Verification items for the finished model (mm, model axes). Face numbers are marked on the shaded views. Round coordinates to 2 decimals unless told otherwise and drop trailing zeros. Loops run counter-clockwise (first coordinate to the right, second up) from the corner with the lowest first, then second, coordinate; pieces in that order, holes last. Notation, with made-up numbers: M -21.5,-28 L 37.5,-28 A20 ccw 37.5,-4 Z; hole C 43.25,12.5 d5. An arc over 180 degrees is marked long. One line per item, written item: value.
Autodesk Inventor part; units mm, degrees
ref_plane "YZ Plane" through (0, 0, 0) normal (1, 0, 0) x (0, 1, 0)
ref_plane "XZ Plane" through (0, 0, 0) normal (0, 1, 0) x (-1, 0, 0)
ref_plane "XY Plane" through (0, 0, 0) normal (0, 0, 1) x (1, 0, 0)
sketch "Sketch1" plane through (0, 0, 0) normal (0, 1, 0) x (-1, 0, 0)
  line L0 (0, 0) -> (114.8965, 0) construction
  line L1 (114.8965, 0) -> (114.8965, -52.636) construction
  line L2 (114.8965, -52.636) -> (0, -52.636) construction
  line L3 (0, -52.636) -> (0, 0) construction
  line L4 (81.8737, -2.7526) -> (21.8737, -2.7526)
  line L5 (21.8737, -2.7526) -> (21.8737, -47.7526)
  line L6 (21.8737, -47.7526) -> (81.8737, -47.7526)
  line L7 (81.8737, -47.7526) -> (81.8737, -2.7526)
  circle A0 centre (76.8737, -7.7526) radius 2
  circle A1 centre (51.8737, -25.2526) radius 6
  circle A2 centre (26.8737, -7.7526) radius 2
  circle A3 centre (76.8737, -42.7526) radius 2
  circle A4 centre (26.8737, -42.7526) radius 2
  circle A5 centre (43.1237, -16.5026) radius 1.5
  circle A6 centre (43.1237, -34.0026) radius 1.5
  circle A7 centre (60.6237, -34.0026) radius 1.5
  circle A8 centre (60.6237, -16.5026) radius 1.5
  point P0 (51.8737, -47.7526)
  dimension "d1" = 60
  dimension "d4" = 45
  dimension "d5" = 4
  dimension "d6" = 5
  dimension "d7" = 5
  dimension "d9" = 12
  dimension "d10" = 22.5
  dimension "d11" = 30
  dimension "d16" = 50
  dimension "d19" = 35
  dimension "d37" = 3
  dimension "d49" = 360
  dimension "d52" = 17.5
extrude "Extrusion1" add sketch "Sketch1" along normal blind 4.5
properties part number "MotorBasePlate"
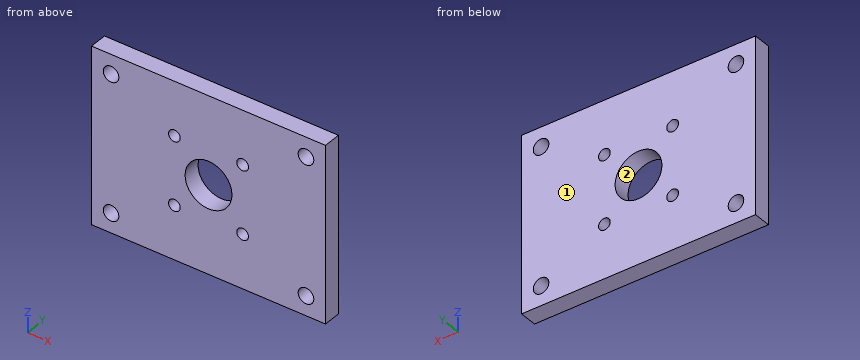
(1) Depth check by flat-ended pin: pin 1 Ø2.5 at (x, z) = (-76.87, -42.75) entering from +Y. Enter the tip coordinate at first touch or a pass-through.
Completed:
pin 1: passes through
(2) Sectioned sample at D-D on x = -28. Enter the section's corners in (y, z).
Completed:
outline: M 0,-47.75 L 4.5,-47.75 L 4.5,-44.41 L 0,-44.41 Z; M 0,-41.1 L 4.5,-41.1 L 4.5,-9.41 L 0,-9.41 Z; M 0,-6.1 L 4.5,-6.1 L 4.5,-2.75 L 0,-2.75 Z
(3) Sectioned sample at C-C on z = -29. Enter the section's corners in (x, y).
Completed:
outline: M -81.87,0 L -56.56,0 L -56.56,4.5 L -81.87,4.5 Z; M -47.19,0 L -21.87,0 L -21.87,4.5 L -47.19,4.5 Z
(4) Sectioned sample at A-A on x = -52. Enter the section's corners in (y, z).
Completed:
outline: M 0,-47.75 L 4.5,-47.75 L 4.5,-31.25 L 0,-31.25 Z; M 0,-19.25 L 4.5,-19.25 L 4.5,-2.75 L 0,-2.75 Z
(5) Sectioned sample at B-B on y = 1.75. Count the separate pieces of the cut face and the enclosed holes in it, and give its area (3 significant figures).
Completed:
separate pieces: 1
enclosed holes: 9
area: 2,510 mm^2
(6) Mould release check, pull along Z, two halves, no side actions. Record for the marked faces 1 and 2: +Z half, -Z half, draft (parallel to the pull), parting line (faces both ways), or undercut.
Completed:
face 1: draft
face 2: undercut
(7) Thickness scan on L1, parallel to X at y = 1.35, z = -16.5; L2, parallel to X at y = 0.95, z = -43; L3, parallel to Z at x = -42, y = 4.2. Record the ranges inside material, lowest first. Write a range as from..to.
Completed:
L1: x = -81.87..-62.12, -59.12..-44.62, -41.62..-21.87
L2: x = -81.87..-78.86, -74.89..-28.86, -24.89..-21.87
L3: z = -47.75..-35, -33.01..-17.5, -15.51..-2.75
